Read the model definition and answer for the solid it produces. Units are mm, in the model's axes. A direction names the side the tool comes from. Give positions to 0.01 mm unless a question says otherwise; leave off trailing zeros. Write each loop counter-clockwise with the first axis right and the second up, starting at its lowest first coordinate (ties: lowest second). Pieces come first, ordered by that corner, then holes. Notation, with made-up numbers: M 86,16 L 94,16 A25 ccw 94,42 Z; hole C 21.25,-1 d3. An arc over 180 degrees is marked long. Write each question's results on one line, items separated by ' | '. Start each with the question number.
Autodesk Inventor part; units mm, degrees
ref_plane "YZ Plane" through (0, 0, 0) normal (1, 0, 0) x (0, 1, 0)
ref_plane "XZ Plane" through (0, 0, 0) normal (0, 1, 0) x (-1, 0, 0)
ref_plane "XY Plane" through (0, 0, 0) normal (0, 0, 1) x (1, 0, 0)
sketch "Sketch1" plane through (0, 0, 0) normal (0, 0, 1) x (1, 0, 0)
  circle A0 centre (0, 0) radius 4.96
  circle A1 centre (0, 0) radius 9.12
  line L0 (-4.96, 0) -> (-4.96, 7.6533)
  line L1 (4.96, 0) -> (4.96, 7.6533)
  dimension "d0" = 9.92
  dimension "d1" = 18.24
extrude "Extrusion1" add sketch "Sketch1" along normal blind 3.18 contours L1 A1 L0 A0 picked at (5.5376, 4.6162)
properties part number "parça6"
Item 1: Section B-B, the plane z = 2.9 is taken. Determine the outline of the cut face in (x, y), then the cut area to 3 significant figures.
Item 2: Section C-C, the plane x = 0 is taken. Determine the outline of the cut face in (y, z).
Item 3: Section D-D, the plane y = 2.5 is taken. Determine the outline of the cut face in (x, z), then the cut area to 3 significant figures.
Item 4: Given P1, Ø1.5, axis at x = 1, z = 0.5, coming from the -Y side, flat-ended and moving along its own axis, determine where the tip first touches the part or whether it passes through.
Item 5: Straight lines are drawn through the part: line 1 (Y direction, x = 0, z = 3); line 2 (X direction, y = 5.5, z = 2.7); line 3 (X direction, y = 5.75, z = 1.4). For each, find the intervals that lie inside material, in ascending order.
Item 6: Determine the mould class of faces 1 (the flat face through (0, -6, 3.18)), 2 (the cylindrical face through (0.11, -4.96, 1.57)) for opening direction X: +X half, -X half, draft (parallel to the pull), parting line (faces both ways), or undercut.
Item 7: For faces 3 (the flat face through (0, -6, 0)), 4 (the flat face through (4.96, 4, 2)), determine the directions among +Z, -Z, +X, -X, +Y, -Y from which every point of the face is accessible in a straight line to the end or side of a thin tool.
Item 8: Section A-A, the plane y = -4 is taken. Determine the outline of the cut face in (x, z), then the cut area to 3 significant figures.
Worked out:
1) outline: M -4.96,0 L -4.96,7.65 A9.12 ccw long 4.96,7.65 L 4.96,0 A4.96 cw Z | area: 137 mm²
2) outline: M -9.12,0 L -4.96,0 L -4.96,3.18 L -9.12,3.18 Z
3) outline: M -8.77,0 L -4.96,0 L -4.96,3.18 L -8.77,3.18 Z; M 4.96,0 L 8.77,0 L 8.77,3.18 L 4.96,3.18 Z | area: 24.2 mm²
4) P1: stops at y = -9.12
5) line 1: y = -9.12 to -4.96 | line 2: x = -7.27 to -4.96, 4.96 to 7.27 | line 3: x = -7.08 to -4.96, 4.96 to 7.08
6) face 1: draft | face 2: undercut
7) face 3: -Z, +X, -X, +Y, -Y | face 4: +Z, -Z, +Y
8) outline: M -8.2,0 L -2.93,0 L -2.93,3.18 L -8.2,3.18 Z; M 2.93,0 L 8.2,0 L 8.2,3.18 L 2.93,3.18 Z | area: 33.5 mm²
